Geometry: final body of the model. Coordinates: model frame, mm. A direction names the side the tool comes from. Give positions to 0.01 mm unless a question says otherwise; leave off trailing zeros. Write each loop counter-clockwise with the first axis right and the second up, starting at its lowest first coordinate (ties: lowest second). Pieces come first, ordered by that corner, then holes.
Q1. Line query: L1, parallel to Y at x = -5, z = 9.5; L2, parallel to Z at x = -16, y = -40; L3, parallel to Y at x = -30.5, z = 17.5. Output: solid intervals per line, ascending.
Q2. Pin query (flat end, axial travel): pin 1 (12 mm diameter, centred on x = -13.5, y = -23.5, fed in from +Z); pin 2 (8 mm diameter, centred on x = -45, y = -5, fed in from +Z); pin 3 (5 mm diameter, centred on x = -5.5, z = 39, fed in from -Y). Return the tip coordinate at first contact, or that it passes through.
Q3. Cut plane C-C on y = -14. Return the cut outline in (x, z), plus the area to 3 significant figures.
Q4. Reachability of faces 4 (the face through (-5, -15, 38)), 5 (the face through (-22, -20, 15)), 6 (the face through (-30, -20, 5)) from +Z, -Z, +X, -X, +Y, -Y: full face, straight path, thin tool, end or side. Return the list, or none.
Q5. Draft query along Y for faces 1 (the face through (-15, -10, 5)), 2 (the face through (-3, -11, 50)), 3 (the face through (-19, -50, 13)). Return one class per face: pulls with the +Y half, pulls with the -Y half, needs draft (parallel to the pull), parting line crosses it, or undercut.
Q6. Cut plane A-A on z = 29.5. Return the cut outline in (x, y).
Q7. Cut plane B-B on x = -7. Return the cut outline in (y, z), plus the area to 4 significant figures.
Q8. Cut plane D-D on y = -35. Return the cut outline in (x, z), plus the area to 3 significant figures.
```python
from build123d import *

# Parameters (mm, degrees)
F1_DEPTH  = 50
F4_DEPTH  = 43
F7_REACH  = 115.9479483752
F11_DEPTH = 35
F12_W     = 20
F12_H     = 10
F14_DEPTH = 30


with BuildPart() as f1:
    # F0 (on Right) → F1 (new body)
    with BuildSketch(Plane.YZ):
        Polygon((-50, 0), (0, 0), (0, 50), (-15, 50), (-15, 25), (-50, 25), align=None)
    extrude(amount=-F1_DEPTH)

    # F2 (on face) → F4 (cut, through all)
    with BuildSketch(Plane.XY.offset(50)):
        Polygon((0, 0), (-50, 0), (-50, -50), (-35, -50), align=None)
    extrude(amount=-F4_DEPTH, mode=Mode.SUBTRACT)

    f7_end = Plane(origin=(-13.8970588235, -19.8529411765, 22.3235294118), x_dir=(-0.5734623444, -0.8192319205, 0), z_dir=(-0.8192319205, 0.5734623444, 0))
    # F6 (on plane+point) → F7 (join, up to a plane its end follows)
    with BuildSketch(Plane.YZ.offset(-50)):
        Polygon((-50, 7), (0, 7), (0, 50), align=None)
    f7_long = extrude(amount=F7_REACH, mode=Mode.PRIVATE)
    add(split(f7_long, bisect_by=f7_end, keep=Keep.TOP, mode=Mode.PRIVATE))

    # F9 (on plane+point) → F11 (cut, through all)
    with BuildSketch(Plane.XY.offset(50)):
        Polygon((0, 0), (-15, 0), (-50, -50), (-35, -50), align=None)
    extrude(amount=-F11_DEPTH, mode=Mode.SUBTRACT)

    # F12 (on face) → F14 (cut, through all)
    with BuildSketch(Plane.YZ):
        with Locations((-20, 5)):
            Rectangle(F12_W, F12_H)
    extrude(amount=-F14_DEPTH, mode=Mode.SUBTRACT)


solid = f1.part
```
Data:
1. L1: y = -50 to -30, -10 to 0
1. L2: z = 0 to 25
1. L3: y = -50 to -43.57, -22.14 to 0
2. pin 1: stops at z = 25
2. pin 2: stops at z = 49.14
2. pin 3: stops at y = -15
3. outline: (-50, 0) - (-30, 0) - (-30, 10) - (0, 10) - (0, 50) - (-9.8, 50) - (-9.8, 15) - (-24.8, 15) - (-24.8, 37.96) - (-50, 37.96) - close
3. area: 1,370 mm2
4. face 4: +Z, +X, -Y
4. face 5: +Z
4. face 6: -Z, +X
5. face 1: undercut
5. face 2: needs draft
5. face 3: pulls with the -Y half
6. outline: (-50, -23.84) - (-31.69, -23.84) - (-15, 0) - (-50, 0) - close; (-10.5, -15) - (0, -15) - (0, 0) - close
7. outline: (-50, 0) - (-30, 0) - (-30, 10) - (-10, 10) - (-10, 0) - (0, 0) - (0, 15) - (-10, 15) - (-10, 50) - (-15, 50) - (-15, 25) - (-50, 25) - close
7. area: 1,075 mm2
8. outline: (-50, 0) - (0, 0) - (0, 25) - (-24.5, 25) - (-24.5, 15) - (-39.5, 15) - (-39.5, 19.9) - (-50, 19.9) - close
8. area: 1,050 mm2
